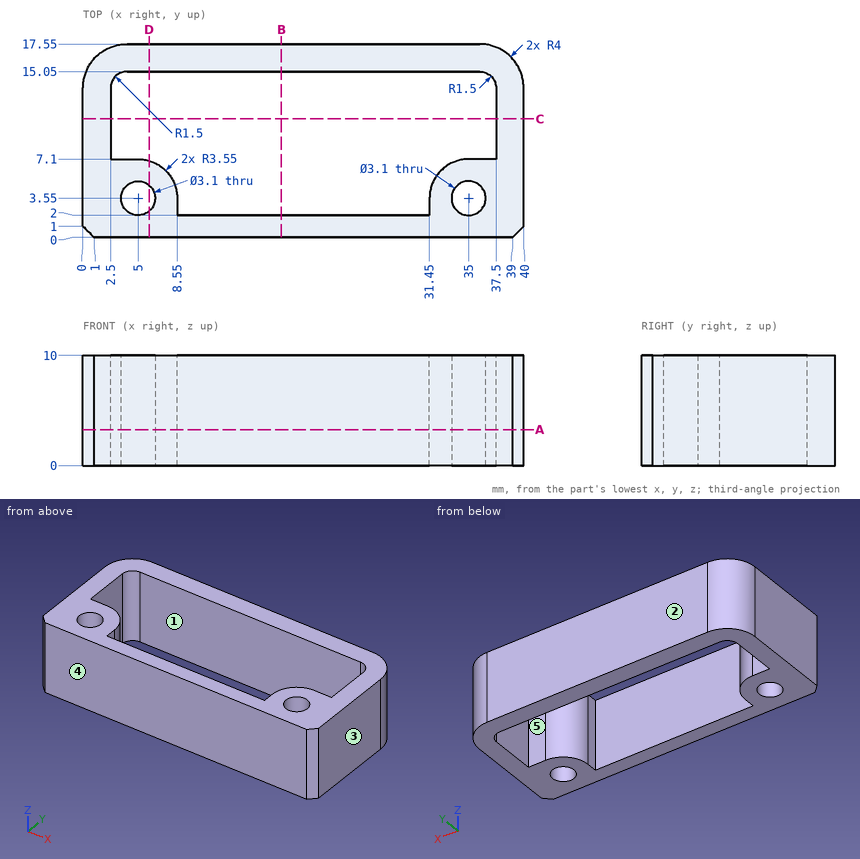
Geometry check sheet. Reference: drawing and pictorial views, mm from the part's lowest x, y, z. A direction names the side the tool comes from. Round coordinates to 2 decimals unless told otherwise and drop trailing zeros. Write each loop counter-clockwise with the first axis right and the second up, starting at its lowest first coordinate (ties: lowest second). Pieces come first, ordered by that corner, then holes.
1. Section check A-A on z = 3.25. Enter the section's corners in (x, y).
2. Access from +Z, -Z, +X, -X, +Y, -Y to the whole of each face (thin tool, end or side, straight path). Record for the marked faces 4 and 5.
3. Section check B-B on x = 18. Enter the section's corners in (y, z).
4. Scan lines: L1, parallel to Y at x = 35, z = 4; L2, parallel to Y at x = 23, z = 4.25; L3, parallel to X at y = 4.5, z = 2.75. Record each from-to range of solid material in increasing order.
5. Section check D-D on x = 6. Enter the section's corners in (y, z).
6. Draft check along Y on the marked faces 1, 2 and 3. Enter one of: +Y half, -Y half, draft (parallel to the pull), parting line (faces both ways), or undercut.
7. Section check C-C on y = 10.75. Enter the section's corners in (x, z), plus the area to 3 significant figures.
Answer:
1. outline: (0, 1) - (1, 0) - (39, 0) - (40, 1) - (40, 13.55) arc R4 ccw to (36, 17.55) - (4, 17.55) arc R4 ccw to (0, 13.55) - close; hole (2.5, 7.1) - (5, 7.1) arc R3.55 cw to (8.55, 3.55) - (8.55, 2) - (31.45, 2) - (31.45, 3.55) arc R3.55 cw to (35, 7.1) - (37.5, 7.1) - (37.5, 13.55) arc R1.5 ccw to (36, 15.05) - (4, 15.05) arc R1.5 ccw to (2.5, 13.55) - close; hole circle Ø3.1 at (5, 3.55); hole circle Ø3.1 at (35, 3.55)
2. face 4: +Z, -Z, +X, -X, -Y
2. face 5: +Z, -Z
3. outline: (0, 0) - (2, 0) - (2, 10) - (0, 10) - close; (15.05, 0) - (17.55, 0) - (17.55, 10) - (15.05, 10) - close
4. L1: y = 0 to 2, 5.1 to 7.1, 15.05 to 17.55
4. L2: y = 0 to 2, 15.05 to 17.55
4. L3: x = 0 to 3.78, 6.22 to 8.42, 31.58 to 33.78, 36.22 to 40
5. outline: (0, 0) - (2.37, 0) - (2.37, 10) - (0, 10) - close; (4.73, 0) - (6.96, 0) - (6.96, 10) - (4.73, 10) - close; (15.05, 0) - (17.55, 0) - (17.55, 10) - (15.05, 10) - close
6. face 1: undercut
6. face 2: +Y half
6. face 3: draft
7. outline: (0, 0) - (2.5, 0) - (2.5, 10) - (0, 10) - close; (37.5, 0) - (40, 0) - (40, 10) - (37.5, 10) - close
7. area: 50.0 mm2
